Work out the finished part from the listing and answer in its coordinate system (mm). A direction names the side the tool comes from. Coordinates: 2 decimals unless noted, no trailing zeros. Order: outer loops, then holes, each group sorted by start corner. A loop starts at its lowest first (then second) coordinate and runs counter-clockwise, first axis right, second up. Notation, with made-up numbers: M -30.75,4 L 25.25,4 A21 cw 25.25,25 Z; hole C -14.5,27.5 d3. An arc over 180 degrees is marked long. Use a Markdown table: item, result.
from build123d import *

# Parameters (mm, degrees)
SKETCH1_W           = 38.1
SKETCH1_H           = 53.975
BOSS_EXTRUDE1_DEPTH = 3.175
SKETCH2_W           = 31.75
SKETCH2_H           = 47.625
BOSS_EXTRUDE2_DEPTH = 1.5875
CHAMFER1_SIZE       = 3.81
SKETCH3_R           = 1.905
CUT_EXTRUDE1_DEPTH  = 1.5875
SKETCH4_R           = 3.96875
CUT_EXTRUDE2_DEPTH  = 125.151898589


with BuildPart() as part:
    # Sketch1 → Boss-Extrude1 (new body)
    with BuildSketch(Plane(origin=(0, 0, 0), x_dir=(1, 0, 0), z_dir=(0, 1, 0))):
        with Locations((-73.117016369, -56.056184953)):
            Rectangle(SKETCH1_W, SKETCH1_H)
    extrude(amount=BOSS_EXTRUDE1_DEPTH)

    # Sketch2 → Boss-Extrude2 (add)
    with BuildSketch(Plane.XZ):
        with Locations((-73.117016369, 56.056184953)):
            Rectangle(SKETCH2_W, SKETCH2_H)
    extrude(amount=BOSS_EXTRUDE2_DEPTH)

    # Chamfer1
    chamfer1_edges = [part.edges().sort_by_distance(p)[0] for p in [
        (-92.167016369, 1.5875, 29.068684953),
        (-54.067016369, 1.5875, 29.068684953),
        (-54.067016369, 1.5875, 83.043684953),
        (-92.167016369, 1.5875, 83.043684953),
    ]]
    chamfer(chamfer1_edges, length=CHAMFER1_SIZE)

    # Sketch3 → Cut-Extrude1 (cut)
    with BuildSketch(Plane(origin=(0, 3.175, 0), x_dir=(1, 0, 0), z_dir=(0, 1, 0))):
        with Locations(Location((-73.117016369, -56.056184953, 0), (0, 0, 270))):
            Circle(SKETCH3_R)
        with BuildLine():
            Line((-74.704516369, -68.656575572), (-74.704516369, -62.204546015))
            ThreePointArc((-74.704516369, -62.204546015), (-79.467016369, -56.056184953), (-74.704516369, -49.907823891))
            Line((-74.704516369, -49.907823891), (-74.704516369, -43.455794334))
            ThreePointArc((-74.704516369, -43.455794334), (-85.817016369, -56.056184953), (-74.704516369, -68.656575572))
        make_face()
        with BuildLine():
            ThreePointArc((-71.529516369, -49.907823891), (-66.767016369, -56.056184953), (-71.529516369, -62.204546015))
            Line((-71.529516369, -62.204546015), (-71.529516369, -68.656575572))
            ThreePointArc((-71.529516369, -68.656575572), (-60.417016369, -56.056184953), (-71.529516369, -43.455794334))
            Line((-71.529516369, -43.455794334), (-71.529516369, -49.907823891))
        make_face()
    extrude(amount=-CUT_EXTRUDE1_DEPTH, mode=Mode.SUBTRACT)

    # Sketch4 → Cut-Extrude2 (cut, through all)
    with BuildSketch(Plane(origin=(0, 3.175, 0), x_dir=(-1, 0, 0), z_dir=(0, 1, 0))):
        with Locations(Location((73.117016369, 56.056184953, 0), (0, 0, 90))):
            Circle(SKETCH4_R)
    extrude(amount=-CUT_EXTRUDE2_DEPTH, mode=Mode.SUBTRACT)


solid = part.part
1. Section D-D on z = 48 is taken. Determine the outline of the cut face in (x, y) (1 decimal).
Answers below:
| item | result |
|---|---|
| outline | M -92.2,0 L -89,0 L -89,-1.6 L -57.2,-1.6 L -57.2,0 L -54.1,0 L -54.1,3.2 L -63.3,3.2 L -63.3,1.6 L -71.5,1.6 L -71.5,3.2 L -74.7,3.2 L -74.7,1.6 L -82.9,1.6 L -82.9,3.2 L -92.2,3.2 Z |
2. Section A-A on z = 40.5 is taken. Determine the outline of the cut face in (x, y) (1 decimal), then the cut area to 3 significant figures.
Answers below:
| item | result |
|---|---|
| outline | M -92.2,0 L -89,0 L -89,-1.6 L -57.2,-1.6 L -57.2,0 L -54.1,0 L -54.1,3.2 L -92.2,3.2 Z |
| area | 171 mm² |
3. Section C-C on x = -62.5 is taken. Determine the outline of the cut face in (y, z) (1 decimal), then the cut area to 3 significant figures.
Answers below:
| item | result |
|---|---|
| outline | M -1.6,32.2 L 0,32.2 L 0,29.1 L 3.2,29.1 L 3.2,49.1 L 1.6,49.1 L 1.6,63 L 3.2,63 L 3.2,83 L 0,83 L 0,79.9 L -1.6,79.9 Z |
| area | 225 mm² |
4. Flat-ended cylindrical pins translate along their axes: P1, Ø3.5, axis at x = -83, z = 58.5, coming from the +Y side; P2, Ø0.8, axis at x = -73.5, y = -1, coming from the +Z side; P3, Ø0.8, axis at x = -66, y = -1, coming from the -Z side. Find the tip coordinate at first contact, or state that the pin passes through.
Answers below:
| item | result |
|---|---|
| P1 | y = 1.59 |
| P2 | z = 79.87 |
| P3 | z = 32.24 |
5. Section B-B on x = -72.5 is taken. Determine the outline of the cut face in (y, z) (1 decimal), then the cut area to 3 significant figures.
Answers below:
| item | result |
|---|---|
| outline | M -1.6,32.2 L 0,32.2 L 0,29.1 L 3.2,29.1 L 3.2,52.1 L -1.6,52.1 Z; M -1.6,60 L 3.2,60 L 3.2,83 L 0,83 L 0,79.9 L -1.6,79.9 Z |
| area | 210 mm² |
6. For a pull along X with two mould halves and no side action, classify faces 6 (the face through (-74.705, 2, 65)), 7 (the face through (-57.242, -1, 56)), 8 (the face through (-90.2, 1.6, 81.2)), 9 (the face through (-71.53, 2, 47)) as +X half, -X half, draft (parallel to the pull), parting line (faces both ways), or undercut.
Answers below:
| item | result |
|---|---|
| face 6 | undercut |
| face 7 | +X half |
| face 8 | -X half |
| face 9 | undercut |
7. Find the intervals of material crossed by probe 1 along X at (y, z) = (-0.7, 44); probe 2 along Y at (x, z) = (-76.5, 81) (3 decimals); probe 3 along Y at (x, z) = (-82, 61), in increasing order.
Answers below:
| item | result |
|---|---|
| probe 1 | -88.99 to -57.24 |
| probe 2 | 0 to 3.175 |
| probe 3 | -1.59 to 1.59 |
8. For faces 1 (the face through (-73, -1.588, 51)), 2 (the face through (-88.992, -1, 56)), 3 (the face through (-73, -1, 32.244)), 4 (the face through (-66.77, 2.39, 55.94)), 5 (the face through (-73, -1, 79.869)), determine the directions among +Z, -Z, +X, -X, +Y, -Y from which every point of the face is accessible in a straight line to the end or side of a thin tool.
Answers below:
| item | result |
|---|---|
| face 1 | +Z, -Z, +X, -X, -Y |
| face 2 | +Z, -Z, -X, -Y |
| face 3 | -Z, +X, -X, -Y |
| face 4 | +Y |
| face 5 | +Z, +X, -X, -Y |
